Verification items for the finished model (mm, model axes). A direction names the side the tool comes from. Round coordinates to 2 decimals unless told otherwise and drop trailing zeros. Write each loop counter-clockwise with the first axis right and the second up, starting at its lowest first coordinate (ties: lowest second). Pieces come first, ordered by that corner, then holes. Notation, with made-up numbers: (40, 59.5) -> (55, 59.5) arc R29 ccw to (55, 87.5) -> close; hole circle Ø4 at (55, 29.25). An arc over 180 degrees is marked (long way). Answer as a JSON object with one key per item and string values. Group by question number.
(1) Gauge pin test, flat ends, axial feed: pin 1 Ø0.8 at (y, z) = (2.5, 0.5) entering from -X; pin 2 Ø1.1 at (y, z) = (3, 0.5) entering from +X. Record the tip position at first contact, or that the pin passes through.
(2) Sectioned sample at A-A on y = 3.75. Record the cut outline in (x, z), and give its area (3 significant figures).
(3) Scan lines: L1, parallel to X at y = 0.85, z = 5; L2, parallel to Z at x = 20, y = 2.75; L3, parallel to Y at x = 16, z = 8.5. Record each from-to range of solid material in increasing order. Write a range as from..to.
(4) Sectioned sample at B-B on z = 5. Record the cut outline in (x, y).
(5) Sectioned sample at C-C on x = 34. Record the cut outline in (y, z).
(6) Draft check along Z on faces 1 (the face through (-36.983, 5.624, 4.89)), 2 (the face through (5, 6.117, 5)), 3 (the face through (5, 5.117, 5)). Enter one of: released by +Z, released by -Z, zero draft, split by the parting line, or undercut.
(7) Set-up check for faces 4 (the face through (5, 3, 9)), 5 (the face through (-30, 5.62, 4.74)): record each of +Z, -Z, +X, -X, +Y, -Y from which the full face is reachable in a straight line by a thin tool's end or side.
```python
from build123d import *

# Parameters (mm, degrees)
SKETCH1_W           = 85.948776221
SKETCH1_H           = 6.116753323
BOSS_EXTRUDE3_DEPTH = 10
FILLET1_RADIUS      = 5
FILLET1_LENGTH      = 6.116753323
FILLET2_RADIUS      = 5
FILLET2_LENGTH      = 6.116753323
SKETCH2_R           = 2
CUT_EXTRUDE1_DEPTH  = 10
SHELL4_START        = -36.984014516
SHELL4_OUTLINE_W    = 4.116753323
SHELL4_OUTLINE_H    = 8
SHELL4_DEPTH        = 85.948776221
SHELL4_START_2      = -36.983829274
SHELL4_2_OUTLINE_W  = 4.116753323
SHELL4_2_OUTLINE_H  = 2
SHELL4_2_DEPTH      = 4.999814758
SHELL4_START_3      = 43.964761705
SHELL4_3_OUTLINE_W  = 4.116753323
SHELL4_3_OUTLINE_H  = 2
SHELL4_3_DEPTH      = 4.999814758


# Read off the part's stored shape, not the designer's step: Shell4
with BuildPart() as part:
    # Sketch1 → Boss-Extrude3 (new body)
    with BuildSketch(Plane.XY):
        with Locations((5.990373594, 3.058376662)):
            Rectangle(SKETCH1_W, SKETCH1_H)
    extrude(amount=BOSS_EXTRUDE3_DEPTH)

    # Fillet1: full round fillet: the end face becomes a half cylinder, R = half its width
    fillet1_face = Plane((48.964761705, 3.058376662, 5), x_dir=(0, -1, 0), z_dir=(1, 0, 0))  # on the end face: x along it, z out of the body
    fillet1_slab = fillet1_face.offset(-FILLET1_RADIUS / 2) * Box(FILLET1_LENGTH, 2 * FILLET1_RADIUS, FILLET1_RADIUS, mode=Mode.PRIVATE)  # the body's end, R deep
    fillet1_round = Plane((43.964761705, 3.058376662, 5), x_dir=(1, 0, 0), z_dir=(0, -1, 0)) * Cylinder(FILLET1_RADIUS, FILLET1_LENGTH, mode=Mode.PRIVATE)  # its axis R under the face
    add(fillet1_slab - fillet1_round, mode=Mode.SUBTRACT)

    # Fillet2: full round fillet: the end face becomes a half cylinder, R = half its width
    fillet2_face = Plane((-36.984014516, 3.058376662, 5), x_dir=(0, 1, 0), z_dir=(-1, 0, 0))  # on the end face: x along it, z out of the body
    fillet2_slab = fillet2_face.offset(-FILLET2_RADIUS / 2) * Box(FILLET2_LENGTH, 2 * FILLET2_RADIUS, FILLET2_RADIUS, mode=Mode.PRIVATE)  # the body's end, R deep
    fillet2_round = Plane((-31.984014516, 3.058376662, 5), x_dir=(-1, 0, 0), z_dir=(0, 1, 0)) * Cylinder(FILLET2_RADIUS, FILLET2_LENGTH, mode=Mode.PRIVATE)  # its axis R under the face
    add(fillet2_slab - fillet2_round, mode=Mode.SUBTRACT)

    # Sketch2 → Cut-Extrude1 (cut)
    with BuildSketch(Plane(origin=(0, 6.116753323, 0), x_dir=(1, 0, 0), z_dir=(0, 1, 0))):
        with Locations(Location((43.964761705, -5, 0), (0, 0, 270))):
            Circle(SKETCH2_R)
        with Locations(Location((-31.984014516, -5, 0), (0, 0, 270))):
            Circle(SKETCH2_R)
    extrude(amount=-CUT_EXTRUDE1_DEPTH, mode=Mode.SUBTRACT)

    # Shell4 outline → Shell4 (cut)
    with BuildSketch(Plane.YZ.offset(SHELL4_START)):
        with Locations((3.058376662, 5)):
            Rectangle(SHELL4_OUTLINE_W, SHELL4_OUTLINE_H)
    extrude(amount=SHELL4_DEPTH, mode=Mode.SUBTRACT)

    # Shell4 2 outline → Shell4 2 (cut)
    with BuildSketch(Plane.YZ.offset(SHELL4_START_2)):
        with Locations((3.058376662, 0)):
            Rectangle(SHELL4_2_OUTLINE_W, SHELL4_2_OUTLINE_H)
        with Locations((3.058376662, 10)):
            Rectangle(SHELL4_2_OUTLINE_W, SHELL4_2_OUTLINE_H)
    extrude(amount=SHELL4_2_DEPTH, mode=Mode.SUBTRACT)

    # Shell4 3 outline → Shell4 3 (cut)
    with BuildSketch(Plane.YZ.offset(SHELL4_START_3)):
        with Locations((3.058376662, 0)):
            Rectangle(SHELL4_3_OUTLINE_W, SHELL4_3_OUTLINE_H)
        with Locations((3.058376662, 10)):
            Rectangle(SHELL4_3_OUTLINE_W, SHELL4_3_OUTLINE_H)
    extrude(amount=SHELL4_3_DEPTH, mode=Mode.SUBTRACT)


solid = part.part
```
Computed values:
{
 "1": {"pin 1": "x = -31.98", "pin 2": "x = 43.96"},
 "2": {"outline": "(-31.98, 0) -> (43.96, 0) -> (43.96, 1) -> (-31.98, 1) -> close; (-31.98, 9) -> (43.96, 9) -> (43.96, 10) -> (-31.98, 10) -> close", "area": "152 mm2"},
 "3": {"L1": "-36.98..-33.98, -29.98..41.96, 45.96..48.96", "L2": "0..1, 9..10", "L3": "0..1, 5.12..6.12"},
 "4": {"outline": "(-36.98, 0) -> (-33.98, 0) -> (-33.98, 1) -> (-36.98, 1) -> close; (-36.98, 5.12) -> (-33.98, 5.12) -> (-33.98, 6.12) -> (-36.98, 6.12) -> close; (-29.98, 0) -> (41.96, 0) -> (41.96, 1) -> (-29.98, 1) -> close; (-29.98, 5.12) -> (41.96, 5.12) -> (41.96, 6.12) -> (-29.98, 6.12) -> close; (45.96, 0) -> (48.96, 0) -> (48.96, 1) -> (45.96, 1) -> close; (45.96, 5.12) -> (48.96, 5.12) -> (48.96, 6.12) -> (45.96, 6.12) -> close"},
 "5": {"outline": "(0, 0) -> (6.12, 0) -> (6.12, 10) -> (0, 10) -> close; hole (1, 1) -> (5.12, 1) -> (5.12, 9) -> (1, 9) -> close"},
 "6": {"face 1": "split by the parting line", "face 2": "zero draft", "face 3": "undercut"},
 "7": {"face 4": "+X, -X", "face 5": "+Y, -Y"}
}
